Geometry: final body of the model. Coordinates: model frame, mm. A direction names the side the tool comes from. Coordinates: 2 decimals unless noted, no trailing zeros. Write each loop counter-clockwise with the first axis right and the second up, starting at its lowest first coordinate (ties: lowest second). Pieces come first, ordered by that corner, then holes.
from build123d import *

# Parameters (mm, degrees)
SKETCH_R        = 5.95
SKETCH_R_2      = 4.5
PAD_DEPTH       = 30
SKETCH001_R     = 10.85
POCKET_DEPTH    = 8
SKETCH002_R     = 10.4
SKETCH002_R_2   = 5
SKETCH002_R_3   = 1.5
POCKET001_DEPTH = 60
SKETCH003_W     = 21
SKETCH003_H     = 21
POCKET002_DEPTH = 20
FILLET_R        = 1


with BuildPart() as part:
    # Sketch → Pad (new body)
    with BuildSketch(Plane.YZ):
        with BuildLine():
            Line((-15, 39.738024), (-15, -45))
            Line((-15, -45), (-15, -64.795761))
            ThreePointArc((-24.587379, -74.38314), (-17.808078, -71.575062), (-15, -64.795761))
            Line((-24.587379, -74.38314), (-30, -74.38314))
            Line((-30, -74.38314), (-30, -124.38314))
            Line((-30, -124.38314), (30, -124.38314))
            Line((30, -124.38314), (30, -74.38314))
            Line((30, -74.38314), (25.005197, -74.38314))
            ThreePointArc((15, -64.377943), (17.930454, -71.452686), (25.005197, -74.38314))
            Line((15, -45), (15, -64.377943))
            Line((15, 31.297371), (15, -45))
            ThreePointArc((15, 31.297371), (14.030328, 34.3011), (11.487377, 36.170874))
            Line((11.487377, 36.170874), (-10.008051, 43.336017))
            ThreePointArc((-10.008051, 43.336017), (-13.424965, 42.814755), (-15, 39.738024))
        make_face()
        with Locations((0, 24.5)):
            Circle(SKETCH_R, mode=Mode.SUBTRACT)
        with Locations((0, -24.5)):
            Circle(SKETCH_R, mode=Mode.SUBTRACT)
        Circle(SKETCH_R_2, mode=Mode.SUBTRACT)
    extrude(amount=PAD_DEPTH)

    # Sketch001 (on Face18 of Pad) → Pocket (cut)
    with BuildSketch(Plane(origin=(0, 0, 0), x_dir=(0, 1, 0), z_dir=(-1, 0, 0))):
        Circle(SKETCH001_R)
    extrude(amount=-POCKET_DEPTH, mode=Mode.SUBTRACT)

    # Sketch002 (on Face16 of Pocket) → Pocket001 (cut)
    with BuildSketch(Plane(origin=(0, -30, 0), x_dir=(0, 0, -1), z_dir=(0, -1, 0))):
        with Locations((89.38314, 15)):
            Circle(SKETCH002_R)
        with Locations((111.38314, 15)):
            Circle(SKETCH002_R_2)
        with Locations((111.38314, 22.5)):
            Circle(SKETCH002_R_3)
        with Locations((103.88314, 15)):
            Circle(SKETCH002_R_3)
        with Locations((111.38314, 7.5)):
            Circle(SKETCH002_R_3)
        with Locations((118.88314, 15)):
            Circle(SKETCH002_R_3)
    extrude(amount=-POCKET001_DEPTH, mode=Mode.SUBTRACT)

    # Sketch003 (on Face16 of Pocket001) → Pocket002 (cut)
    with BuildSketch(Plane(origin=(0, -30, 0), x_dir=(0, 0, -1), z_dir=(0, -1, 0))):
        with Locations((111.38314, 15)):
            Rectangle(SKETCH003_W, SKETCH003_H)
    extrude(amount=-POCKET002_DEPTH, mode=Mode.SUBTRACT)

    # Fillet
    fillet_edges = [part.edges().sort_by_distance(p)[0] for p in [
        (15, -30, -74.38314),
        (15, 30, -74.38314),
    ]]
    fillet(fillet_edges, radius=FILLET_R)


solid = part.part
Item 1: Material intervals for probe 1 along Z at (x, y) = (19, -17.5); probe 2 along X at (y, z) = (-16, -105); probe 3 along Y at (x, z) = (16, 0), sorted ascending.
Derived:
probe 1: z = -124.38 to -121.88, -100.88 to -98.98, -79.78 to -71.25
probe 2: x = 0 to 4.5, 25.5 to 30
probe 3: y = -15 to -4.5, 4.5 to 15
Item 2: Section A-A, the plane y = 0. State how many separate pieces and enclosed holes the cut face has, plus the area to 3 significant figures.
Derived:
separate pieces: 4
enclosed holes: 6
area: 3,400 mm2
Item 3: Set-up query: faces 4 (the flat face through (15, 15, -16)), 5 (the flat face through (15, -27, -74.383)), 6 (the flat face through (15, -20, -121.883)), 7 (the cylindrical face through (15.457, -0.42, -78.993)), 8 (the flat face through (8, 5, 0)). Return all of +Z, -Z, +X, -X, +Y, -Y with unobstructed straight access to the full face (end or side cutting, diameter ignored); none if empty.
Derived:
face 4: +Z, +X, -X, +Y
face 5: +Z, +X, -X, -Y
face 6: -Y
face 7: +Y, -Y
face 8: -X
Item 4: Pin query (flat end, axial travel): pin 1 (8 mm diameter, centred on x = 7, y = 3.5, fed in from +Z); pin 2 (5 mm diameter, centred on x = 16, y = -27, fed in from +Z); pin 3 (5 mm diameter, centred on x = 4, z = 3.5, fed in from +Y). Return the tip coordinate at first contact, or that it passes through.
Derived:
pin 1: stops at z = 40.17
pin 2: stops at z = -74.38
pin 3: stops at y = 15
Item 5: Section D-D, the plane y = -13. Output: boundary loops of the cut face in (x, z).
Derived:
outline: (0, -124.38) - (30, -124.38) - (30, 43.08) - (0, 43.08) - close; hole (4.5, -121.88) - (25.5, -121.88) - (25.5, -100.88) - (4.5, -100.88) - close; hole circle Ø20.8 at (15, -89.38)
Item 6: Pull-direction query (Z, two-part tool) for faces 1 (the cylindrical face through (14.79, 14.06, 34.26)), 2 (the flat face through (15, -15, -12)), 3 (the flat face through (4.5, -20, -111)); classes: released by +Z, released by -Z, zero draft, split by the parting line, or undercut.
Derived:
face 1: released by +Z
face 2: zero draft
face 3: undercut
Item 7: Section B-B, the plane z = 0. Output: boundary loops of the cut face in (x, y).
Derived:
outline: (0, -15) - (30, -15) - (30, -4.5) - (8, -4.5) - (8, -10.85) - (0, -10.85) - close; (0, 10.85) - (8, 10.85) - (8, 4.5) - (30, 4.5) - (30, 15) - (0, 15) - close
